Here's how the part is built. I have some questions about the finished solid (model axes, mm). A direction names the side the tool comes from. Coordinates: 2 decimals unless noted, no trailing zeros. Write each loop counter-clockwise with the first axis right and the second up, starting at its lowest first coordinate (ties: lowest second). Pieces come first, ordered by that corner, then holes. Notation, with made-up numbers: (-10, -10) - (4, -10) arc R16 ccw to (4, 8) - close; hole circle Ø4 at (80.25, -32). An arc over 180 degrees is marked (long way). Answer in a Markdown table with one row per item. Add a question column.
Item 1: Imagine slicing it at B-B (x = 0). Please give me the cut outline in (y, z), plus the area to 3 significant figures.
Item 2: If I drill on probe 1 along X at (y, z) = (20.5, 0); probe 2 along Y at (x, z) = (-32, 51); probe 3 along X at (y, z) = (25, -51), over which ranges is the centre line in solid material (lowest first)? Write a range as from..to.
Item 3: Which directions (+Z, -Z, +X, -X, +Y, -Y) give clear straight access to the entire face, cutting with the end or side of a thin tool? Please do faces 5 (the face through (11.75, 12, 7)), 6 (the face through (1, 0, -1)).
Item 4: Imagine slicing it at A-A (y = 12). Please give me the cut outline in (x, z), plus the area to 3 significant figures.
Item 5: We'd pull the mould along Z, two halves only. Please class faces 1 (the face through (38, 40, -82)), 2 (the face through (30.04, 19.72, 95.38)), 3 (the face through (-32, 12, 0)), 4 (the face through (-34.471, 22.745, 83.137)): +Z half, -Z half, draft (parallel to the pull), parting line (faces both ways), or undercut.
Item 6: Imagine slicing it at D-D (x = -47.5). Please give me the cut outline in (y, z), plus the area to 3 significant figures.
Item 7: I'm going to push flat-ended pins straight in: pin 1 (7.5 mm diameter, centred on x = -5, y = 15, fed in from -Z); pin 2 (10 mm diameter, centred on y = 34.5, z = 58.5, fed in from -X); pin 3 (7 mm diameter, centred on y = 12.5, z = -10, fed in from +X); pin 4 (6 mm diameter, centred on x = -11, z = 26, fed in from -Y). Where does each tip first touch, or does it pass through?
Item 8: Imagine slicing it at C-C (z = 0). Please give me the cut outline in (x, y).
from build123d import *

# Parameters (mm, degrees)
SKETCH1_R           = 100
BOSS_EXTRUDE1_DEPTH = 40
SKETCH2_R           = 90
CUT_EXTRUDE1_DEPTH  = 35
SKETCH3_W           = 46.75
SKETCH3_H           = 26.5
BOSS_EXTRUDE2_DEPTH = 15
SKETCH4_W           = 3
SKETCH4_H           = 9
CUT_EXTRUDE2_DEPTH  = 15


with BuildPart() as part:
    # Sketch1 → Boss-Extrude1 (new body)
    with BuildSketch(Plane(origin=(0, 0, 0), x_dir=(1, 0, 0), z_dir=(0, 1, 0))):
        with Locations(Location((0, 0, 0), (0, 0, 270))):
            Circle(SKETCH1_R)
    extrude(amount=BOSS_EXTRUDE1_DEPTH)

    # Sketch2 → Cut-Extrude1 (cut)
    with BuildSketch(Plane(origin=(0, 40, 0), x_dir=(1, 0, 0), z_dir=(0, 1, 0))):
        with Locations(Location((0, 0, 0), (0, 0, 270))):
            Circle(SKETCH2_R)
    extrude(amount=-CUT_EXTRUDE1_DEPTH, mode=Mode.SUBTRACT)

    # Sketch3 → Boss-Extrude2 (add)
    with BuildSketch(Plane(origin=(0, 5, 0), x_dir=(1, 0, 0), z_dir=(0, 1, 0))):
        with Locations((-8.625, 0)):
            Rectangle(SKETCH3_W, SKETCH3_H)
        Polygon((0, 10.25), (11.75, 10.25), (11.75, -10.25), (0, -10.25), (-29, -10.25), (-29, 10.25), align=None, mode=Mode.SUBTRACT)
    extrude(amount=BOSS_EXTRUDE2_DEPTH)

    # Sketch4 → Cut-Extrude2 (cut)
    with BuildSketch(Plane(origin=(0, 20, 0), x_dir=(1, 0, 0), z_dir=(0, 1, 0))):
        with Locations((13.25, 0)):
            Rectangle(SKETCH4_W, SKETCH4_H)
    extrude(amount=-CUT_EXTRUDE2_DEPTH, mode=Mode.SUBTRACT)


solid = part.part
Here are the results:
| question | item | result |
|---|---|---|
| 1 | outline | (0, -100) - (40, -100) - (40, -90) - (5, -90) - (5, -13.25) - (20, -13.25) - (20, -10.25) - (5, -10.25) - (5, 10.25) - (20, 10.25) - (20, 13.25) - (5, 13.25) - (5, 90) - (40, 90) - (40, 100) - (0, 100) - close |
| 1 | area | 1,790 mm2 |
| 2 | probe 1 | x = -100..-90, 90..100 |
| 2 | probe 2 | y = 0..5 |
| 2 | probe 3 | x = -86.02..-74.16, 74.16..86.02 |
| 3 | face 5 | +Y |
| 3 | face 6 | +Z, -Z, +X, -X, -Y |
| 4 | outline | circle Ø200 at (0, 0); (-32, -13.25) - (14.75, -13.25) - (14.75, -4.5) - (11.75, -4.5) - (11.75, -10.25) - (-29, -10.25) - (-29, 10.25) - (11.75, 10.25) - (11.75, 4.5) - (14.75, 4.5) - (14.75, 13.25) - (-32, 13.25) - close; hole circle Ø180 at (0, 0) |
| 4 | area | 6,350 mm2 |
| 5 | face 1 | draft |
| 5 | face 2 | parting line |
| 5 | face 3 | undercut |
| 5 | face 4 | undercut |
| 6 | outline | (0, -88) - (40, -88) - (40, -76.44) - (5, -76.44) - (5, 76.44) - (40, 76.44) - (40, 88) - (0, 88) - close |
| 6 | area | 1,690 mm2 |
| 7 | pin 1 | stops at z = -99.99 |
| 7 | pin 2 | stops at x = -84.49 |
| 7 | pin 3 | stops at x = 99.79 |
| 7 | pin 4 | stops at y = 0 |
| 8 | outline | (-100, 0) - (100, 0) - (100, 40) - (90, 40) - (90, 5) - (-29, 5) - (-29, 20) - (-32, 20) - (-32, 5) - (-90, 5) - (-90, 40) - (-100, 40) - close |
